from build123d import *

# Parameters (mm, degrees)
SKETCH1_R           = 6.5
BOSS_EXTRUDE1_DEPTH = 7
BOSS_EXTRUDE2_DEPTH = 2.5
SKETCH3_R           = 1.25
CUT_EXTRUDE1_DEPTH  = 17.888639434
SKETCH4_R           = 1.25
CUT_EXTRUDE2_DEPTH  = 17.888639434
FILLET1_R           = 1.5
SKETCH5_R           = 4.45
CUT_EXTRUDE3_DEPTH  = 2


with BuildPart() as part:
    # Sketch1 → Boss-Extrude1 (new body)
    with BuildSketch(Plane(origin=(0, 0, 0), x_dir=(1, 0, 0), z_dir=(0, 1, 0))):
        Circle(SKETCH1_R)
        with BuildLine():
            Line((-3.95, 2.049390153), (-3.95, -2.049390153))
            ThreePointArc((-3.95, -2.049390153), (0, -4.45), (3.95, -2.049390153))
            Line((3.95, -2.049390153), (3.95, 2.049390153))
            ThreePointArc((3.95, 2.049390153), (0, 4.45), (-3.95, 2.049390153))
        make_face(mode=Mode.SUBTRACT)
    extrude(amount=BOSS_EXTRUDE1_DEPTH)

    # Sketch2 → Boss-Extrude2 (add, symmetric)
    with BuildSketch(Plane.XY):
        Polygon((5.5, 7), (5.5, 0), (6.5, 0), (8.132076804, 3.5), (13.029353969, 1.216362154), (13.45197223, 2.122669941), (8.554695065, 4.406307787), (9.188622458, 5.765769468), (14.085899623, 3.482131621), (14.740957929, 4.886908691), (10.209418994, 7), align=None)
        Polygon((-5.5, 0), (-5.5, 7), (-6.5, 7), (-8.132076804, 3.5), (-13.029353969, 5.783637846), (-13.45197223, 4.877330059), (-8.554695065, 2.593692213), (-9.188622458, 1.234230532), (-14.085899623, 3.517868379), (-14.740957929, 2.113091309), (-10.209418994, 0), align=None)
    extrude(amount=BOSS_EXTRUDE2_DEPTH, both=True)

    # Sketch3 → Cut-Extrude1 (cut, through all)
    with BuildSketch(Plane(origin=(4.504621032, 9.660190978, 0), x_dir=(0.906307787, -0.422618262, 0), z_dir=(0.422618262, 0.906307787, 0))):
        with Locations((8.794548103, 0)):
            Circle(SKETCH3_R)
    extrude(amount=-CUT_EXTRUDE1_DEPTH, mode=Mode.SUBTRACT)

    # Sketch4 → Cut-Extrude2 (cut, through all)
    with BuildSketch(Plane(origin=(-1.823465481, -3.910434344, 0), x_dir=(0.906307787, -0.422618262, 0), z_dir=(-0.422618262, -0.906307787, 0))):
        with Locations((-11.752875935, 0)):
            Circle(SKETCH4_R)
    extrude(amount=-CUT_EXTRUDE2_DEPTH, mode=Mode.SUBTRACT)

    # Fillet1
    fillet1_edges = [part.edges().sort_by_distance(p)[0] for p in [
        (13.2406631, 1.669516047, 2.5),
        (14.413428776, 4.184520156, 2.5),
        (10.209418994, 7, 0),
        (13.2406631, 1.669516047, -2.5),
        (14.413428776, 4.184520156, -2.5),
        (-13.2406631, 5.330483953, 2.5),
        (-14.413428776, 2.815479844, 2.5),
        (-14.413428776, 2.815479844, -2.5),
        (-10.209418994, 0, 0),
        (-13.2406631, 5.330483953, -2.5),
    ]]
    fillet(fillet1_edges, radius=FILLET1_R)

    # Sketch5 → Cut-Extrude3 (cut)
    with BuildSketch(Plane(origin=(0, 7, 0), x_dir=(1, 0, 0), z_dir=(0, 1, 0))):
        Circle(SKETCH5_R)
    extrude(amount=-CUT_EXTRUDE3_DEPTH, mode=Mode.SUBTRACT)


solid = part.part
Read the model definition and answer for the solid it produces. Units are mm, in the model's axes. A direction names the side the tool comes from. Round coordinates to 2 decimals unless told otherwise and drop trailing zeros. Write each loop counter-clockwise with the first axis right and the second up, starting at its lowest first coordinate (ties: lowest second). Pieces come first, ordered by that corner, then holes.
Q1. Straight lines are drawn through the part: line 1 (X direction, y = 4.5, z = 2.25); line 2 (X direction, y = 3.25, z = -1.5); line 3 (Z direction, x = 3.5, y = 6.5). For each, find the intervals that lie inside material, in ascending order.
Values:
line 1: x = -12.64 to -10.28, -7.67 to -3.84, 3.84 to 8.6, 11.9 to 13.82
line 2: x = -14.12 to -13.51, -9.96 to -3.95, 3.95 to 8.02, 8.67 to 11.03
line 3: z = -5.48 to -2.75, 2.75 to 5.48
Q2. Find section C-C on z = 3.75. Determine the outline of the cut face in (x, y).
Values:
outline: (-5.31, 0) - (-2.4, 0) - (-2.4, 7) - (-5.31, 7) - close; (2.4, 0) - (5.31, 0) - (5.31, 7) - (2.4, 7) - close
Q3. Flat-ended cylindrical pins translate along their axes: P1, Ø3.5, axis at x = -10.5, y = 3.5, coming from the -Z side; P2, Ø4, axis at y = 3, z = -5, coming from the +X side; P3, Ø1.5, axis at x = 9.5, y = 4, coming from the +Z side. Find the tip coordinate at first contact, or state that the pin passes through.
Values:
P1: stops at z = -2.5
P2: stops at x = 5.77
P3: stops at z = 2.5
Q4. The mould has two halves that part along Y. Classify faces 5 (the face through (14.01, 4.38, -2.07)), 6 (the face through (-9.949, 3.244, -0.521)), 7 (the face through (5, 7, 0)), 8 (the face through (-9, 3, -2.5)): released by +Y, released by -Y, zero draft, split by the parting line, or undercut.
Values:
face 5: released by -Y
face 6: undercut
face 7: released by +Y
face 8: zero draft
Q5. Find section B-B on z = 1.75. Determine the outline of the cut face in (x, y), and give its area (3 significant figures).
Values:
outline: (-14.56, 2.03) - (-10.51, 0.14) arc R1.5 ccw to (-9.88, 0) - (-3.95, 0) - (-3.95, 5) - (-4.09, 5) - (-4.09, 7) - (-6.5, 7) - (-8.13, 3.5) - (-12.85, 5.7) - (-13.27, 4.79) - (-8.55, 2.59) - (-9.19, 1.23) - (-13.9, 3.43) - close; (3.95, 0) - (6.5, 0) - (8.13, 3.5) - (12.85, 1.3) - (13.27, 2.21) - (8.55, 4.41) - (9.19, 5.77) - (13.9, 3.57) - (14.56, 4.97) - (10.51, 6.86) arc R1.5 ccw to (9.88, 7) - (4.09, 7) - (4.09, 5) - (3.95, 5) - close
area: 84.4 mm2
Q6. Find section A-A on x = 3.25. Determine the outline of the cut face in (y, z).
Values:
outline: (0, -5.63) - (7, -5.63) - (7, -3.04) - (0, -3.04) - close; (0, 3.04) - (7, 3.04) - (7, 5.63) - (0, 5.63) - close
Q7. A tool of negligible diameter and unlimited length cuts with its end or side. For faces 1 (the face through (-3.95, 2, 0)), 2 (the face through (8.87, 5.08, -0.04)), 3 (the face through (-9.46, 4.12, 0.04)), 4 (the face through (-9, 3, 2.5)), from which of +Z, -Z, +X, -X, +Y, -Y can it reach the whole face along a straight path? Write none if from no direction.
Values:
face 1: +Y, -Y
face 2: +Z, -Z
face 3: +Z, -Z, +Y
face 4: +Z, -X, +Y, -Y
